from build123d import *

# Parameters (mm, degrees)
EXTRUDE_1_DEPTH     = 9
CUT_EXTRUDE_START   = -5
CUT_EXTRUDE_1_DEPTH = 5
SKETCH_12_W         = 2.5
SKETCH_12_H         = 7
CUT_EXTRUDE_3_DEPTH = 42.911887352
FILLET_11_R         = 2
FILLET_1_R          = 1
SKETCH_10_W         = 8
SKETCH_10_H         = 4
EXTRUDE_3_DEPTH     = 2
FILLET_5_R          = 5
FILLET_10_R         = 7.5
FILLET_14_R         = 2
FILLET_15_R         = 1.5
FILLET_16_R         = 2
FILLET_17_R         = 1
FILLET_18_R         = 2
SKETCH_11_R         = 5.1
CUT_EXTRUDE_2_DEPTH = 44.514365603


# Some blends are built 0.0001 mm under size
with BuildPart() as part:
    # Эскиз2 → Бобышка-Вытянуть1 (new body)
    with BuildSketch(Plane.XY):
        with BuildLine():
            Line((-18, 0), (-15, 0))
            Line((-15, 0), (-15, 7))
            Line((-15, 7), (-10, 7))
            Line((-10, 7), (-10, 0))
            ThreePointArc((-10, 0), (-7.39984978, -6.726233956), (-0.951555354, -9.954624172))
            ThreePointArc((-0.951555354, -9.954624172), (10.407523967, -15.498539394), (15.320888862, -27.144247806))
            ThreePointArc((15.320888862, -27.144247806), (8.452365235, -21.873844259), (0, -20))
            ThreePointArc((0, -20), (-1.44344914, -20.176216472), (-2.802111775, -20.69451514))
            ThreePointArc((-2.802111775, -20.69451514), (-7.346697493, -22.426064476), (-12.174852362, -23.009539415))
            ThreePointArc((-12.174852362, -23.009539415), (-16.488233618, -23.738589268), (-20.315570084, -25.857142338))
            ThreePointArc((-20.315570084, -25.857142338), (-31.05163084, -24.430323259), (-29.168151763, -13.764896883))
            ThreePointArc((-29.168151763, -13.764896883), (-22.544234788, -7.726123715), (-18, 0))
        make_face()
    extrude(amount=EXTRUDE_1_DEPTH)

    # Эскиз6 → Вырез-Вытянуть1 (cut)
    with BuildSketch(Plane.XY.offset(9).offset(CUT_EXTRUDE_START)):
        with BuildLine():
            ThreePointArc((-9.55, -2.96605799), (-16.390256677, -12.316180922), (-16.898984287, -23.890078556))
            ThreePointArc((-16.898984287, -23.890078556), (-14.577958647, -23.229625817), (-12.174852362, -23.009539415))
            ThreePointArc((-12.174852362, -23.009539415), (-7.346697493, -22.426064476), (-2.802111775, -20.69451514))
            ThreePointArc((-2.802111775, -20.69451514), (-1.44344914, -20.176216472), (0, -20))
            ThreePointArc((0, -20), (8.452365235, -21.873844259), (15.320888862, -27.144247806))
            ThreePointArc((15.320888862, -27.144247806), (10.407523967, -15.498539394), (-0.951555354, -9.954624172))
            ThreePointArc((-0.951555354, -9.954624172), (-6.307192762, -7.760110789), (-9.55, -2.96605799))
        make_face()
    extrude(amount=CUT_EXTRUDE_1_DEPTH, mode=Mode.SUBTRACT)

    # Эскиз12 → Вырез-Вытянуть3 (cut, through all)
    with BuildSketch(Plane.ZY.offset(15)):
        with Locations((1.25, 3.5)):
            Rectangle(SKETCH_12_W, SKETCH_12_H)
        with Locations((7.75, 3.5)):
            Rectangle(SKETCH_12_W, SKETCH_12_H)
    extrude(amount=-CUT_EXTRUDE_3_DEPTH, mode=Mode.SUBTRACT)

    # Скругление11
    fillet_11_edges = [part.edges().sort_by_distance(p)[0] for p in [
        (-10, 0, 7.75),
        (-10, 0, 1.25),
    ]]
    fillet(fillet_11_edges, radius=FILLET_11_R)

    # Скругление1
    fillet_1_edges = [part.edges().sort_by_distance(p)[0] for p in [
        (15.320888862, -27.144247806, 2),
    ]]
    fillet(fillet_1_edges, radius=FILLET_1_R)

    # Эскиз10 → Бобышка-Вытянуть3 (add)
    with BuildSketch(Plane(origin=(0, 7, 0), x_dir=(-1, 0, 0), z_dir=(0, 1, 0))):
        with Locations((14, 4.5)):
            Rectangle(SKETCH_10_W, SKETCH_10_H)
    extrude(amount=EXTRUDE_3_DEPTH)

    # Скругление5
    fillet_5_edges = [part.edges().sort_by_distance(p)[0] for p in [
        (-10, 9, 4.5),
    ]]
    fillet(fillet_5_edges, radius=FILLET_5_R)

    # Скругление10
    fillet_10_edges = [part.edges().sort_by_distance(p)[0] for p in [
        (-16.898984287, -23.890078556, 6.5),
    ]]
    fillet(fillet_10_edges, radius=FILLET_10_R - 0.0001)  # a hair under: the kernel refuses the full size

    # Скругление14
    fillet_14_edges = [part.edges().sort_by_distance(p)[0] for p in [
        (-15, 7, 4.5),
    ]]
    fillet(fillet_14_edges, radius=FILLET_14_R)

    # Скругление15
    fillet_15_edges = [part.edges().sort_by_distance(p)[0] for p in [
        (-17.5, 7, 6.5),
        (-15, 2.5, 6.5),
        (-17.5, 7, 2.5),
        (-15.585786438, 6.414213562, 2.5),
        (-15.585786438, 6.414213562, 6.5),
        (-15, 2.5, 2.5),
    ]]
    fillet(fillet_15_edges, radius=FILLET_15_R)

    # Скругление16
    # the kernel refuses this fillet: 2 mm, written as the material it adds along each edge
    with BuildSketch(Plane(origin=(-11.832159566, -2, 6.5), x_dir=(-0.6907726827654878, -0.7230719886325089, 0), z_dir=(-0.7230719886325089, 0.6907726827654878, 0))) as fillet_16_piece_1_section:
        with BuildLine():
            CenterArc((2 + FILLET_16_R, FILLET_16_R), FILLET_16_R, 180, 90)
            Line((2, FILLET_16_R), (2, 0))
            Line((2, 0), (2 + FILLET_16_R, 0))
        make_face()
    fillet_16_piece_1 = revolve(axis=Axis((-11.832159566, -2, 6.5), (0, 0, 1)), revolution_arc=223.691304566, mode=Mode.PRIVATE)
    fillet_16_piece_1 = split(fillet_16_piece_1, bisect_by=Plane(origin=(-9.962064569, 0, 7.231915875), z_dir=(0, -1, 0)), keep=Keep.TOP, mode=Mode.PRIVATE)
    fillet_16_piece_1 = fillet_16_piece_1 - Plane(origin=(0, 0, 7.231915875), x_dir=(-1, 0, 0), z_dir=(0, 0, -1)) * Cylinder(10, 17, mode=Mode.PRIVATE)
    fillet_16_piece_1 = fillet_16_piece_1 - Plane(origin=(2.479707116, -18.943734501, 7.231915875), x_dir=(-0.6014853558135568, 0.7988838255602869, 0), z_dir=(0, 0, -1)) * Cylinder(20, 17, mode=Mode.PRIVATE)
    add(fillet_16_piece_1)
    with BuildSketch(Plane(origin=(-11.832159566, -2, 6.5), x_dir=(-0.6907726827654878, -0.7230719886325089, 0), z_dir=(-0.7230719886325089, 0.6907726827654878, 0))) as fillet_16_piece_2_section:
        with BuildLine():
            CenterArc((2 + FILLET_16_R, FILLET_16_R), FILLET_16_R, 180, 90)
            Line((2, FILLET_16_R), (2, 0))
            Line((2, 0), (2 + FILLET_16_R, 0))
        make_face()
    fillet_16_piece_2 = revolve(axis=Axis((-11.832159566, -2, 6.5), (0, 0, 1)), revolution_arc=223.691304566, mode=Mode.PRIVATE)
    fillet_16_piece_2 = split(fillet_16_piece_2, bisect_by=Plane(origin=(-11.088968436, 0, 6.841402023), z_dir=(0, 1, 0)), keep=Keep.TOP, mode=Mode.PRIVATE)
    fillet_16_piece_2 = split(fillet_16_piece_2, bisect_by=Plane(origin=(-10, 0.441530369, 6.841402023), z_dir=(-1, 0, 0)), keep=Keep.TOP, mode=Mode.PRIVATE)
    add(fillet_16_piece_2)
    with BuildSketch(Plane(origin=(-13.5, 0, 6.5), x_dir=(0, 0, 1), z_dir=(1, 0, 0))) as fillet_16_piece_3:
        with BuildLine():
            CenterArc((FILLET_16_R, -FILLET_16_R), FILLET_16_R, 90, 90)
            Line((0, -FILLET_16_R), (0, 0))
            Line((0, 0), (FILLET_16_R, 0))
        make_face()
    extrude(amount=1.667840434)
    with BuildSketch(Plane(origin=(-11.832159566, -2, 2.5), x_dir=(-0.6907726827654875, -0.7230719886325091, 0), z_dir=(-0.7230719886325091, 0.6907726827654875, 0))) as fillet_16_piece_4_section:
        with BuildLine():
            CenterArc((2 + FILLET_16_R, -FILLET_16_R), FILLET_16_R, 90, 90)
            Line((2, -FILLET_16_R), (2, 0))
            Line((2, 0), (2 + FILLET_16_R, 0))
        make_face()
    fillet_16_piece_4 = revolve(axis=Axis((-11.832159566, -2, 2.5), (0, 0, 1)), revolution_arc=223.691304566, mode=Mode.PRIVATE)
    fillet_16_piece_4 = split(fillet_16_piece_4, bisect_by=Plane(origin=(-9.962064569, 0, 1.768084125), z_dir=(0, -1, 0)), keep=Keep.TOP, mode=Mode.PRIVATE)
    fillet_16_piece_4 = fillet_16_piece_4 - Plane(origin=(0, 0, 1.768084125), x_dir=(-1, 0, 0), z_dir=(0, 0, -1)) * Cylinder(10, 17, mode=Mode.PRIVATE)
    add(fillet_16_piece_4)
    with BuildSketch(Plane(origin=(-11.832159566, -2, 2.5), x_dir=(-0.6907726827654875, -0.7230719886325091, 0), z_dir=(-0.7230719886325091, 0.6907726827654875, 0))) as fillet_16_piece_5_section:
        with BuildLine():
            CenterArc((2 + FILLET_16_R, -FILLET_16_R), FILLET_16_R, 90, 90)
            Line((2, -FILLET_16_R), (2, 0))
            Line((2, 0), (2 + FILLET_16_R, 0))
        make_face()
    fillet_16_piece_5 = revolve(axis=Axis((-11.832159566, -2, 2.5), (0, 0, 1)), revolution_arc=223.691304566, mode=Mode.PRIVATE)
    fillet_16_piece_5 = split(fillet_16_piece_5, bisect_by=Plane(origin=(-10, 0.441530341, 2.15859789), z_dir=(-1, 0, 0)), keep=Keep.TOP, mode=Mode.PRIVATE)
    add(fillet_16_piece_5)
    with BuildSketch(Plane(origin=(-13.5, 0, 2.5), x_dir=(0, 0, -1), z_dir=(1, 0, 0))) as fillet_16_piece_6:
        with BuildLine():
            CenterArc((FILLET_16_R, FILLET_16_R), FILLET_16_R, 180, 90)
            Line((0, FILLET_16_R), (0, 0))
            Line((0, 0), (FILLET_16_R, 0))
        make_face()
    extrude(amount=1.667840434)
    with BuildSketch(Plane(origin=(-13.5, 0, 4), x_dir=(0, 0, -1), z_dir=(1, 0, 0))) as fillet_16_piece_7:
        with BuildLine():
            CenterArc((1.5 + FILLET_16_R, FILLET_16_R), FILLET_16_R, 180, 90)
            Line((1.5 + FILLET_16_R, 0), (1.5, 0))
            Line((1.5, 0), (1.5, FILLET_16_R))
        make_face()
    revolve(axis=Axis((-13.5, 0, 4), (0, 1, 0)), revolution_arc=90)
    with BuildSketch(Plane(origin=(-15, 0, 4), x_dir=(0, 1, 0), z_dir=(0, 0, 1))) as fillet_16_piece_8:
        with BuildLine():
            CenterArc((FILLET_16_R, FILLET_16_R), FILLET_16_R, 180, 90)
            Line((0, FILLET_16_R), (0, 0))
            Line((0, 0), (FILLET_16_R, 0))
        make_face()
    extrude(amount=1)
    with BuildSketch(Plane(origin=(-13.5, 0, 5), x_dir=(0, 0, 1), z_dir=(1, 0, 0))) as fillet_16_piece_9:
        with BuildLine():
            CenterArc((1.5 + FILLET_16_R, -FILLET_16_R), FILLET_16_R, 90, 90)
            Line((1.5 + FILLET_16_R, 0), (1.5, 0))
            Line((1.5, 0), (1.5, -FILLET_16_R))
        make_face()
    revolve(axis=Axis((-13.5, 0, 5), (0, -1, 0)), revolution_arc=90)

    # Скругление17
    fillet_17_edges = [part.edges().sort_by_distance(p)[0] for p in [
        (-18, 8.75, 2.5),
        (-18, 7.439339828, 2.939339828),
        (-18, 7, 4.5),
        (-18, 8.75, 6.5),
        (-18, 7.439339828, 6.060660172),
    ]]
    fillet(fillet_17_edges, radius=FILLET_17_R - 0.0001)  # a hair under: the kernel refuses the full size

    # Скругление18
    fillet_18_edges = [part.edges().sort_by_distance(p)[0] for p in [
        (-9.55, -2.96605799, 5.25),
    ]]
    fillet(fillet_18_edges, radius=FILLET_18_R)

    # Эскиз11 → Вырез-Вытянуть2 (cut, through all)
    with BuildSketch(Plane.XY.offset(9)):
        with Locations((-25, -20)):
            Circle(SKETCH_11_R)
    extrude(amount=-CUT_EXTRUDE_2_DEPTH, mode=Mode.SUBTRACT)


solid = part.part
Input: part model. Units: mm. Frame: model coordinates. A direction names the side the tool comes from. Give positions to 0.01 mm unless a question says otherwise; leave off trailing zeros. Loops run counter-clockwise (first coordinate to the right, second up) from the corner with the lowest first, then second, coordinate; pieces in that order, holes last. Notation, with made-up numbers: (6.25, -24) - (30.25, -24) arc R12 cw to (30.25, -2) - close; hole circle Ø6 at (69.5, -32.5). An arc over 180 degrees is marked (long way). Use CSV: the item, a comma, the result in double quotes. Start each with the question number.
Item 1: Mould query, pull axis Y, two halves, no side actions, for faces 4 (the cylindrical face through (7.207, -21.343, 1.972)), 5 (the cylindrical face through (-14.57, 3.52, 6.05)), 6 (the flat face through (-16, 9, 5)). Classes: pulls with the +Y half, pulls with the -Y half, needs draft (parallel to the pull), parting line crosses it, or undercut.
Item 2: Reachability of faces 1 (the flat face through (-3, -16, 4)), 2 (the cylindrical face through (-15.6, 6.43, 4.51)), 3 (the cylindrical face through (-14.55, 3.52, 2.93)) from +Z, -Z, +X, -X, +Y, -Y: full face, straight path, thin tool, end or side. Return the list, or none.
Item 3: Section D-D on x = 9. Return loops of the section in (y, z).
Item 4: Line query: line 1 (X direction, y = -17, z = 8.25); line 2 (Y direction, x = -20.5, z = 3.5); line 3 (Y direction, x = -27, z = 1.25). Output: solid intervals per line, ascending.
Item 5: Section B-B on y = -13. Return loops of the section in (x, z), then the cut area to 3 significant figures.
Item 6: Contact query for flat-ended pins moving along their axis: P1, Ø5, axis at y = -12, z = 4.5, coming from the -X side; P2, Ø2, axis at x = -13, y = 6, coming from the -Z side; P3, Ø3, axis at y = 2.5, z = 3.5, coming from the +X side; P4, Ø1, axis at x = 5.5, z = 6, coming from the +Y side. Output: stop coordinate, or through.
Item 7: Section A-A on x = -21. Return loops of the section in (y, z).
Item 8: Section C-C on y = -22.5. State how many separate pieces and enclosed holes the cut face has, then the cut area to 3 significant figures.
Ans:
1,face 4,"pulls with the -Y half"
1,face 5,"undercut"
1,face 6,"pulls with the +Y half"
2,face 1,"+Z, +X, -Y"
2,face 2,"+Z, -Z, -X"
2,face 3,"-Z, -X"
3,outline,"(-22.14, 0) - (-14.16, 0) - (-14.16, 4) - (-22.14, 4) - close"
4,line 1,"x = -31.87 to -29.12, -20.88 to -17.43"
4,line 2,"y = -26 to -22.4, -17.6 to -4.88"
4,line 3,"y = -27.23 to -24.69, -15.31 to -12.17"
5,outline,"(-28.08, 0) - (7.47, 0) - (7.47, 4) - (-16.62, 4) - (-16.62, 9) - (-28.08, 9) - close"
5,area,"200 mm2"
6,P1,"stops at x = -30.1"
6,P2,"stops at z = 2.5"
6,P3,"stops at x = -10"
6,P4,"passes through"
7,outline,"(-26.34, 0) - (-23.16, 0) - (-23.16, 9) - (-26.34, 9) - close; (-16.84, 0) - (-5.65, 0) - (-5.65, 9) - (-16.84, 9) - close"
8,separate pieces,"3"
8,enclosed holes,"0"
8,area,"108 mm2"
